Could you check a few things on this model? Use its own coordinates, in mm. Face numbers are marked on the shaded views. Give positions to 0.01 mm unless a question says otherwise; leave off trailing zeros. Loops run counter-clockwise (first coordinate to the right, second up) from the corner with the lowest first, then second, coordinate; pieces in that order, holes last. Notation, with made-up numbers: M 18,89 L 51,89 A24 cw 51,113 Z; hole C -2,44 d1. An arc over 180 degrees is marked long. Use a Markdown table: item, result. Add a question column.
1) We'd pull the mould along Z, two halves only. Please class the marked faces 1, 2, 3 and 4: +Z half, -Z half, draft (parallel to the pull), parting line (faces both ways), or undercut.
2) Suppose I cut it at C-C on z = 0.5. List the corners of the cut face in (x, y) for me.
3) Suppose I cut it at B-B on x = -6. List the corners of the cut face in (y, z) for me, and give its area (3 significant figures).
4) If I drill on line 1 along Y through (x, z) = (-7, 1.5); line 2 along Z through (x, y) = (-6, 4.15); line 3 along X through (y, z) = (10.5, 5.25), over which ranges is the centre line in solid material (lowest first)? Write a range as [from, to].
5) Will these pins go through, and if not, where does the flat tip stop? pin 1 Ø1 at (y, z) = (8, 2) entering from -X; pin 2 Ø3 at (y, z) = (-3, 1.5) entering from -X; pin 3 Ø2 at (x, z) = (-5.5, 4) entering from +Y; pin 4 Ø1.5 at (x, y) = (-3.5, -1) entering from +Z.
```python
from build123d import *

# Parameters (mm, degrees)
F1_DEPTH    = 6.8
F2_R        = 3.39999
F3_R        = 1.55
F4_DEPTH    = 24.001
F3_R_2      = 2.05
F5_DEPTH    = 7
F0_W        = 8
F0_H        = 24
F6_DEPTH    = 6.8
F7_T1_DEPTH = 7
F8_T1_DEPTH = 91.4331581264


# Not quite as in the source:
# - a fillet or chamfer that OpenCascade refuses, or shapes differently, is made with other operations: its cross-section is extruded or revolved along the edge and cut away or added
# - a fillet or chamfer is up to 0.001 mm smaller than in the source, because OpenCascade refuses the exact size
# - a feature names something its author has since deleted; it is built from what else it names


with BuildPart() as f1:
    # F0 (on Top) → F1 (new body)
    with BuildSketch(Plane.XY):
        Polygon((-2, -12), (0, -12), (0, 12), (-2, 12), (-9, 12), (-9, 3.5), (-2, 3.5), (-2, -3.5), (-9, -3.5), (-9, -12), align=None)
    extrude(amount=F1_DEPTH)

    # F2 (radius 3.4 in the source; OpenCascade refuses exactly that, so slightly less here)
    f2_edges = [f1.edges().sort_by_distance(p)[0] for p in [
        (-9, 7.75, 6.8),
        (-9, 7.75, 0),
        (-9, -7.75, 0),
        (-9, -7.75, 6.8),
    ]]
    fillet(f2_edges, radius=F2_R)

    # F3 (on face) → F4 (cut, through all)
    with BuildSketch(Plane(origin=(0, 12, 0), x_dir=(-1, 0, 0), z_dir=(0, 1, 0))):
        with Locations((6, 3.4)):
            Circle(F3_R)
    extrude(amount=-F4_DEPTH, mode=Mode.SUBTRACT)

    # F3 (on face) → F5 (cut)
    with BuildSketch(Plane(origin=(0, 12, 0), x_dir=(-1, 0, 0), z_dir=(0, 1, 0))):
        with Locations((6, 3.4)):
            Circle(F3_R_2)
        with Locations((6, 3.4)):
            Circle(F3_R, mode=Mode.SUBTRACT)
    extrude(amount=-F5_DEPTH, mode=Mode.SUBTRACT)

    # F0 (on Top) → F6 (join, through all)
    with BuildSketch(Plane.XY):
        with Locations((4, 0)):
            Rectangle(F0_W, F0_H)
    extrude(amount=F6_DEPTH)

    # F7: fillet of radius 7 on 1 edges, made by hand

    # F7_s2 → F7_t1 (cut)
    with BuildSketch(Plane.XZ.offset(-3.5)):
        with BuildLine():
            ThreePointArc((-2.0003998352, 6.7999885178), (0.1189410708, 1.9796991069), (4.9980806884, -0.0004))
            Line((4.9980806884, -0.0004), (4.9980806884, -0.7005365685))
            ThreePointArc((4.9980806884, -0.7005365685), (1.4990403442, -0.7001365685), (-2, -0.7001365685))
            Line((-2, -0.7001365685), (-2.7001365685, 0))
            ThreePointArc((-2.7001365685, 0), (-2.7001365685, 3.3999942589), (-2.7002478875, 6.7798908011))
            Line((-2.7002478875, 6.7798908011), (-2.0003998352, 6.7999885178))
        make_face()
    extrude(amount=F7_T1_DEPTH, mode=Mode.SUBTRACT)

    # F8: chamfer of 5 x 13 on 1 edges, made by hand

    # F8_s2 → F8_t1 (cut)
    with BuildSketch(Plane.XZ.offset(-45.7165790632)):
        Polygon((8, 5), (-5, 0), (8, 0), align=None)
    extrude(amount=F8_T1_DEPTH, mode=Mode.SUBTRACT)


solid = f1.part
```
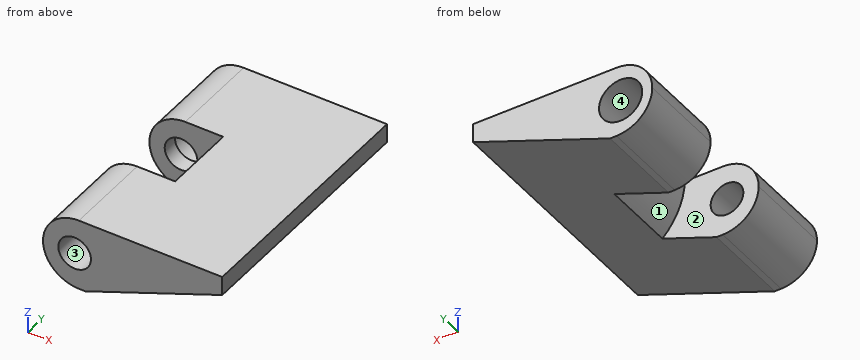
Answer block:
| question | item | result |
|---|---|---|
| 1 | face 1 | -Z half |
| 1 | face 2 | draft |
| 1 | face 3 | undercut |
| 1 | face 4 | undercut |
| 2 | outline | M -7.37,-12 L -3.7,-12 L -3.7,-3.5 L -7.37,-3.5 Z; M -7.37,3.5 L -3.7,3.5 L -3.7,12 L -7.37,12 Z |
| 3 | outline | M -12,0.02 L -3.5,0.02 L -3.5,1.85 L -12,1.85 Z; M -12,4.95 L -3.5,4.95 L -3.5,6.78 L -12,6.78 Z; M 3.5,0.02 L 12,0.02 L 12,1.35 L 5,1.35 L 5,1.85 L 3.5,1.85 Z; M 3.5,4.95 L 5,4.95 L 5,5.45 L 12,5.45 L 12,6.78 L 3.5,6.78 Z |
| 3 | area | 55.1 mm^2 |
| 4 | line 1 | y = [-12, -3.5], [3.5, 12] |
| 4 | line 2 | z = [0.02, 1.85], [4.95, 6.78] |
| 4 | line 3 | x = [-8.45, -6.88], [-5.12, 8] |
| 5 | pin 1 | stops at x = -8.88 |
| 5 | pin 2 | stops at x = -8.97 |
| 5 | pin 3 | stops at y = 5 |
| 5 | pin 4 | passes through |
